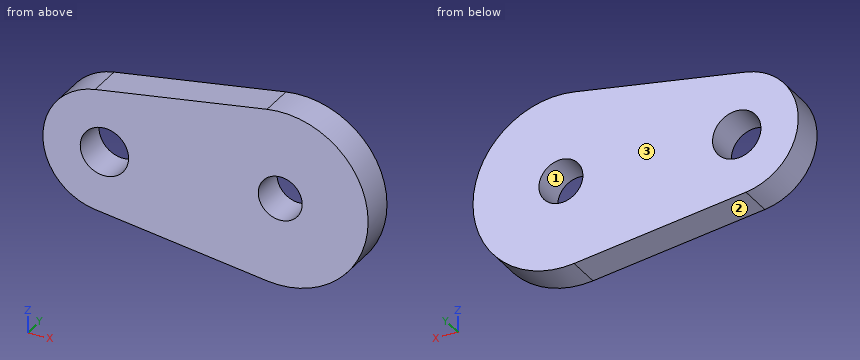
from build123d import *

# Parameters (mm, degrees)
SKETCH1_R           = 7
SKETCH1_R_2         = 2.75
SKETCH1_R_3         = 10
SKETCH1_R_4         = 2.5
BOSS_EXTRUDE1_DEPTH = 4


with BuildPart() as part:
    # Sketch1 → Boss-Extrude1 (new body)
    # profile 1 of 3: a face of its own
    with BuildSketch(Plane(origin=(0, 0, 0), x_dir=(1, 0, 0), z_dir=(0, 1, 0))):
        Circle(SKETCH1_R)
        with Locations(Location((0, 0, 0), (0, 0, 270))):
            Circle(SKETCH1_R_2, mode=Mode.SUBTRACT)
    # profile 2 of 3: a face of its own
    with BuildSketch(Plane(origin=(0, 0, 0), x_dir=(1, 0, 0), z_dir=(0, 1, 0))):
        with BuildLine():
            ThreePointArc((18.5, -9.886859967), (10, 0), (18.5, 9.886859967))
            Line((18.5, 9.886859967), (-1.05, 6.920801977))
            ThreePointArc((-1.05, 6.920801977), (4.563441684, 5.308012811), (7, 0))
            ThreePointArc((7, 0), (4.563441684, -5.308012811), (-1.05, -6.920801977))
            Line((-1.05, -6.920801977), (18.5, -9.886859967))
        make_face()
    # profile 3 of 3: a face of its own
    with BuildSketch(Plane(origin=(0, 0, 0), x_dir=(1, 0, 0), z_dir=(0, 1, 0))):
        with Locations((20, 0)):
            Circle(SKETCH1_R_3)
        with Locations(Location((20, 0, 0), (0, 0, 270))):
            Circle(SKETCH1_R_4, mode=Mode.SUBTRACT)
    extrude(amount=BOSS_EXTRUDE1_DEPTH)


solid = part.part
Could you check a few things on this model? Use its own coordinates, in mm. Face numbers are marked on the shaded views. Give positions to 0.01 mm unless a question says otherwise; leave off trailing zeros. Order: outer loops, then holes, each group sorted by start corner. A loop starts at its lowest first (then second) coordinate and runs counter-clockwise, first axis right, second up.
1. I need wall thicknesses on L1, parallel to X at y = 2.55, z = 0; L2, parallel to X at y = 2.6, z = 1.5; L3, parallel to Z at x = 1.5, y = 2.2. Which ranges of each line are inside material? Lowest first, please.
2. Suppose I cut it at C-C (y = 3.1). List the corners of the cut face in (x, z) for me.
3. Suppose I cut it at A-A (x = 20). List the corners of the cut face in (y, z) for me, plus the area to 3 significant figures.
4. Will this pin go through, and if not, where does the flat tip stop? P1, Ø1.5, axis at x = 21.5, y = 2.5, coming from the +Z side.
5. Suppose I cut it at B-B (z = 0). List the corners of the cut face in (x, y) for me.
6. Suppose I cut it at D-D (x = 0). List the corners of the cut face in (y, z) for me, plus the area to 3 significant figures.
7. We'd pull the mould along X, two halves only. Please class the marked faces 1, 2 and 3: pulls with the +X half, pulls with the -X half, needs draft (parallel to the pull), parting line crosses it, or undercut.
Solved:
1. L1: x = -7 to -2.75, 2.75 to 17.5, 22.5 to 30
1. L2: x = -6.84 to -2.3, 2.3 to 18, 22 to 29.89
1. L3: z = -7.31 to -2.3, 2.3 to 7.31
2. outline: (-1.05, -6.92) - (18.5, -9.89) arc R10 ccw (long way) to (18.5, 9.89) - (-1.05, 6.92) arc R7 ccw to start; hole circle Ø5.5 at (0, 0); hole circle Ø5 at (20, 0)
3. outline: (0, -10) - (4, -10) - (4, -2.5) - (0, -2.5) - close; (0, 2.5) - (4, 2.5) - (4, 10) - (0, 10) - close
3. area: 60.0 mm2
4. P1: stops at z = 9.97
5. outline: (-7, 0) - (-2.75, 0) - (-2.75, 4) - (-7, 4) - close; (2.75, 0) - (17.5, 0) - (17.5, 4) - (2.75, 4) - close; (22.5, 0) - (30, 0) - (30, 4) - (22.5, 4) - close
6. outline: (0, -7.08) - (4, -7.08) - (4, -2.75) - (0, -2.75) - close; (0, 2.75) - (4, 2.75) - (4, 7.08) - (0, 7.08) - close
6. area: 34.6 mm2
7. face 1: undercut
7. face 2: pulls with the -X half
7. face 3: needs draft
